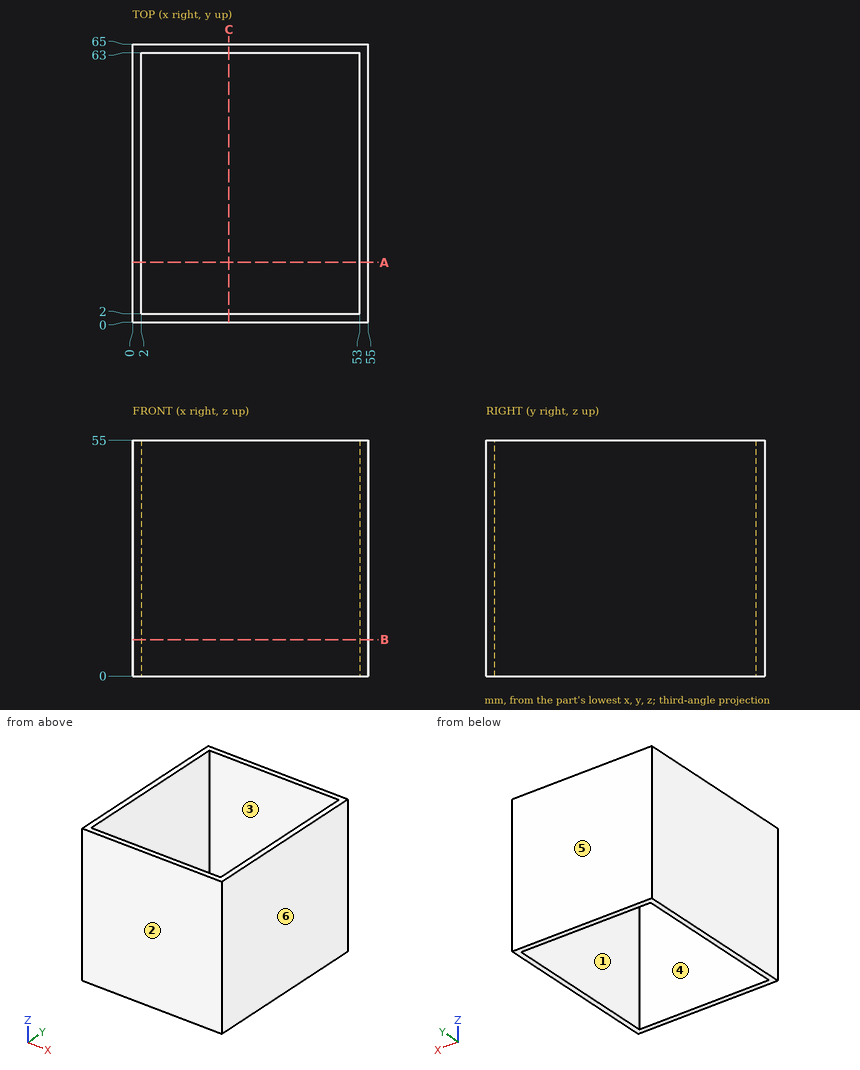
Geometry check sheet. Reference: drawing and pictorial views, mm from the part's lowest x, y, z. A direction names the side the tool comes from. Round coordinates to 2 decimals unless told otherwise and drop trailing zeros. Order: outer loops, then holes, each group sorted by start corner. A loop starts at its lowest first (then second) coordinate and runs counter-clockwise, first axis right, second up. Notation, with made-up numbers: (18.25, -31.75) -> (23.25, -31.75) arc R33 cw to (23.25, 7.25) -> close; hole circle Ø7 at (60, 28). An arc over 180 degrees is marked (long way). One line per item, written item: value. Start each with the question number.
Q1. Mould release check, pull along X, two halves, no side actions. Record for the marked faces 3, 4, 5 and 6: pulls with the +X half, pulls with the -X half, needs draft (parallel to the pull), parting line crosses it, or undercut.
Q2. Cross-section at C-C (x = 22.5). Record the boundary of the cut face in (y, z), and give its area (3 significant figures).
Q3. Thickness scan on line 1 (Y direction, x = 42, z = 24); line 2 (X direction, y = 62.5, z = 50). Record the ranges inside material, lowest first.
Q4. Set-up check for the marked faces 1 and 2: record each of +Z, -Z, +X, -X, +Y, -Y from which the full face is reachable in a straight line by a thin tool's end or side.
Q5. Cross-section at A-A (y = 14). Record the boundary of the cut face in (x, z), and give its area (3 significant figures).
Q6. Cross-section at B-B (z = 8.5). Record the boundary of the cut face in (x, y), and give its area (3 significant figures).
Completed:
1. face 3: undercut
1. face 4: undercut
1. face 5: needs draft
1. face 6: pulls with the +X half
2. outline: (0, 0) -> (2, 0) -> (2, 55) -> (0, 55) -> close; (63, 0) -> (65, 0) -> (65, 55) -> (63, 55) -> close
2. area: 220 mm²
3. line 1: y = 0 to 2, 63 to 65
3. line 2: x = 0 to 2, 53 to 55
4. face 1: +Z, -Z
4. face 2: +Z, -Z, +X, -X, -Y
5. outline: (0, 0) -> (2, 0) -> (2, 55) -> (0, 55) -> close; (53, 0) -> (55, 0) -> (55, 55) -> (53, 55) -> close
5. area: 220 mm²
6. outline: (0, 0) -> (55, 0) -> (55, 65) -> (0, 65) -> close; hole (2, 2) -> (53, 2) -> (53, 63) -> (2, 63) -> close
6. area: 464 mm²
